Read the model definition and answer for the solid it produces. Units are mm, in the model's axes. A direction names the side the tool comes from. Give positions to 0.01 mm unless a question says otherwise; leave off trailing zeros. Order: outer loops, then holes, each group sorted by start corner. A loop starts at its lowest first (then second) coordinate and runs counter-clockwise, first axis right, second up. Notation, with made-up numbers: (20, -19) - (31, -19) arc R18 ccw to (31, 9) - close; hole circle Ø6 at (87, 24.25). An arc over 180 degrees is marked (long way). Return JSON: item names as keys, results as strings.
```python
from build123d import *

# Parameters (mm, degrees)
SKETCH1_R               = 2.54
BOSS_EXTRUDE1_DEPTH     = 6.35
CUT_EXTRUDE1_DEPTH      = 5.334
CUT_EXTRUDE1_DEPTH_BACK = 5.334
CUT_EXTRUDE2_DEPTH      = 5.334
CUT_EXTRUDE2_DEPTH_BACK = 5.334
SKETCH6_R               = 5.334
CUT_EXTRUDE3_DEPTH      = 7.35
CHAMFER1_SIZE           = 0.635


with BuildPart() as part:
    # Sketch1 → Boss-Extrude1 (new body)
    with BuildSketch(Plane(origin=(0, 0, 0), x_dir=(1, 0, 0), z_dir=(0, 1, 0))):
        Polygon((0, 33.02), (0, 0), (22.86, 0), (106.700989027, 0), (106.700989027, 38.586695169), (106.700989027, 56.366695169), (106.700989027, 86.36), (20.32, 86.36), (0, 86.36), (0, 53.34), align=None)
        with Locations((14.605, 43.18)):
            Circle(SKETCH1_R, mode=Mode.SUBTRACT)
        with Locations((94.039183737, 48.746695169)):
            Circle(SKETCH1_R, mode=Mode.SUBTRACT)
    extrude(amount=BOSS_EXTRUDE1_DEPTH)

    # Sketch4 → Cut-Extrude1 (cut, two sides)
    with BuildSketch(Plane.ZY.offset(-14.605)) as cut_extrude1_sk:
        Polygon((-46.28, 2.68), (-40.08, 2.68), (-37.68, 5.08), (-37.68, 6.35), (-48.68, 6.35), (-48.68, 5.08), align=None)
    extrude(amount=CUT_EXTRUDE1_DEPTH, mode=Mode.SUBTRACT)
    extrude(cut_extrude1_sk.sketch, amount=-CUT_EXTRUDE1_DEPTH_BACK, mode=Mode.SUBTRACT)

    # Sketch5 → Cut-Extrude2 (cut, two sides)
    with BuildSketch(Plane.XY.offset(-48.746695169)) as cut_extrude2_sk:
        Polygon((90.939183737, 2.68), (97.139183737, 2.68), (99.539183737, 5.08), (99.539183737, 6.35), (88.539183737, 6.35), (88.539183737, 5.08), align=None)
    extrude(amount=CUT_EXTRUDE2_DEPTH, mode=Mode.SUBTRACT)
    extrude(cut_extrude2_sk.sketch, amount=-CUT_EXTRUDE2_DEPTH_BACK, mode=Mode.SUBTRACT)

    # Sketch6 → Cut-Extrude3 (cut, through all)
    with BuildSketch(Plane.XZ):
        with Locations((12.7, -8.89)):
            Circle(SKETCH6_R)
        with Locations((73.680989027, -48.746695169)):
            Circle(SKETCH6_R)
        with Locations((12.7, -77.47)):
            Circle(SKETCH6_R)
    extrude(amount=-CUT_EXTRUDE3_DEPTH, mode=Mode.SUBTRACT)

    # Chamfer1
    chamfer1_edges = [part.edges().sort_by_distance(p)[0] for p in [
        (7.366, 6.35, -8.89),
        (68.346989027, 6.35, -48.746695169),
        (7.366, 6.35, -77.47),
    ]]
    chamfer(chamfer1_edges, length=CHAMFER1_SIZE)


solid = part.part
```
Q1. A cutting plane is placed at B-B (y = 1.25). Write down the section's boundary in (x, z) (3 decimals), and give its area (3 significant figures).
Values:
{"outline": "(0, -86.36) - (106.701, -86.36) - (106.701, 0) - (0, 0) - close; hole circle Ø10.668 at (12.7, -77.47); hole circle Ø10.668 at (12.7, -8.89); hole circle Ø5.08 at (14.605, -43.18); hole circle Ø10.668 at (73.681, -48.747); hole circle Ø5.08 at (94.039, -48.747)", "area": "8,910 mm²"}
Q2. Consider L1, parallel to X at y = 3, z = -48.5; L2, parallel to X at y = 3.75, z = -49.5; L3, parallel to X at y = 4.75, z = -48. Determine where each line is inside the solid, lowest interval first.
Values:
{"L1": "x = 0 to 68.35, 79.01 to 90.62, 97.46 to 106.7", "L2": "x = 0 to 68.4, 78.96 to 89.87, 98.21 to 106.7", "L3": "x = 0 to 9.27, 19.94 to 68.4, 78.96 to 88.87, 99.21 to 106.7"}
Q3. For faces 1 (the cylindrical face through (15.97, 1.32, -45.32)), 2 (the flat face through (14.68, 3.86, -38.9)), determine the directions among +Z, -Z, +X, -X, +Y, -Y from which every point of the face is accessible in a straight line to the end or side of a thin tool.
Values:
{"face 1": "+Y, -Y", "face 2": "+Y"}
Q4. A cutting plane is placed at A-A (z = -8.89). Write down the section's boundary in (x, y) (3 decimals), and give its area (3 significant figures).
Values:
{"outline": "(0, 0) - (7.366, 0) - (7.366, 5.715) - (6.731, 6.35) - (0, 6.35) - close; (18.034, 0) - (106.701, 0) - (106.701, 6.35) - (18.669, 6.35) - (18.034, 5.715) - close", "area": "609 mm²"}
Q5. Given pin 1 (8 mm diameter, centred on x = 94.04, z = -48.75, fed in from +Y); pin 2 (6.5 mm diameter, centred on x = 12.7, z = -8.89, fed in from -Y); pin 3 (1.5 mm diameter, centred on x = 11, z = -40, fed in from +Y), each flat-ended and moving along its own axis, determine where each tip first touches the part or whether it passes through.
Values:
{"pin 1": "stops at y = 3.58", "pin 2": "passes through", "pin 3": "stops at y = 3.51"}
Q6. Determine the mould class of faces 3 (the flat face through (54, 3, -86.36)), 4 (the flat face through (106.701, 3, -43)), 5 (the flat face through (19.939, 5, -43)) for opening direction Z: released by +Z, released by -Z, zero draft, split by the parting line, or undercut.
Values:
{"face 3": "released by -Z", "face 4": "zero draft", "face 5": "undercut"}
